Check sheet for the modelled part. Datum: model origin and axes. Units: mm. A direction names the side the tool comes from. Round coordinates to 2 decimals unless told otherwise and drop trailing zeros. Loops run counter-clockwise (first coordinate to the right, second up) from the corner with the lowest first, then second, coordinate; pieces in that order, holes last. Notation, with made-up numbers: (-33, 87.25) - (-15, 87.25) arc R17 cw to (-15, 119.25) - close; hole circle Ø11 at (-4.5, 17.25). An arc over 180 degrees is marked (long way). Put each result on its own line as item: value. Start each with the question number.
Item 1: Tool access check on faces 1 (the cylindrical face through (-0.65, -2.93, 26.32)), 2 (the flat face through (0, 3.998, 49)), 3 (the flat face through (-1, 3, 49)). Record the directions out of +Z, -Z, +X, -X, +Y, -Y that give a thin tool (end or side, any length) a straight path to the whole face; none if there is none.
Item 2: Section check D-D, the plane y = -2. Record the cut outline in (x, z).
Item 3: Section check B-B, the plane y = 0. Record the cut outline in (x, z).
Item 4: Section check C-C, the plane z = 11. Record the cut outline in (x, y).
Item 5: Gauge pin test, flat ends, axial feed: pin 1 Ø0.9 at (y, z) = (3.5, 47.5) entering from +X; pin 2 Ø2 at (y, z) = (1.5, 36.5) entering from -X; pin 3 Ø0.6 at (x, z) = (-0.5, 50) entering from +Y; pin 4 Ø2.5 at (x, y) = (0.5, 0.5) entering from -Z. Record the tip position at first contact, or that the pin passes through.
Item 6: Section check A-A, the plane x = 0. Record the cut outline in (y, z), and give its area (3 significant figures).
Item 7: Material ranges on line 1 along Z through (x, y) = (3.75, -1.5); line 2 along Y through (x, z) = (0, 31.5); line 3 along Y through (x, z) = (1.5, 5), recorded low to high.
from build123d import *

# Parameters (mm, degrees)
SKETCH1_R           = 3
BOSS_EXTRUDE1_DEPTH = 53.38
SKETCH2_W           = 2
SKETCH2_H           = 1.17
BOSS_EXTRUDE2_DEPTH = 9.16
SKETCH3_R           = 4.25
BOSS_EXTRUDE3_DEPTH = 2


with BuildPart() as part:
    # Sketch1 → Boss-Extrude1 (new body)
    with BuildSketch(Plane.XY):
        Circle(SKETCH1_R)
    extrude(amount=BOSS_EXTRUDE1_DEPTH)

    # Sketch2 → Boss-Extrude2 (add)
    with BuildSketch(Plane.XY.offset(53.38)):
        with Locations((0, 3.413427125)):
            Rectangle(SKETCH2_W, SKETCH2_H)
    extrude(amount=-BOSS_EXTRUDE2_DEPTH)

    # Sketch3 → Boss-Extrude3 (add)
    with BuildSketch(Plane.XY.offset(53.38)):
        Circle(SKETCH3_R)
    extrude(amount=BOSS_EXTRUDE3_DEPTH)


solid = part.part
Check result:
1. face 1: -Z
1. face 2: -Z, +X, -X, +Y
1. face 3: -Z, -X, +Y
2. outline: (-3.75, 53.38) - (-2.24, 53.38) - (-2.24, 0) - (2.24, 0) - (2.24, 53.38) - (3.75, 53.38) - (3.75, 55.38) - (-3.75, 55.38) - close
3. outline: (-4.25, 53.38) - (-3, 53.38) - (-3, 0) - (3, 0) - (3, 53.38) - (4.25, 53.38) - (4.25, 55.38) - (-4.25, 55.38) - close
4. outline: circle Ø6 at (0, 0)
5. pin 1: x = 1
5. pin 2: x = -2.96
5. pin 3: y = 4
5. pin 4: z = 0
6. outline: (-4.25, 53.38) - (-3, 53.38) - (-3, 0) - (3, 0) - (3, 44.22) - (4, 44.22) - (4, 53.38) - (4.25, 53.38) - (4.25, 55.38) - (-4.25, 55.38) - close
6. area: 346 mm²
7. line 1: 53.38 to 55.38
7. line 2: -3 to 3
7. line 3: -2.6 to 2.6
